from build123d import *

# Parameters (mm, degrees)
F0_R     = 3.175
F0_R_2   = 3.1994548284
F0_R_3   = 14.2875
F0_R_4   = 2.413
F0_R_5   = 13.97
F1_DEPTH = 6.35
F2_R     = 5.08


# Not quite as in the source:
# - a length typed as a fraction of an inch, garbled in the dataset ("3 / 203.2 mm" for 3/8 in), is restored


with BuildPart() as f1:
    # F0 (on Top) → F1 (new body)
    with BuildSketch(Plane.XY):
        Polygon((570.0438245296, 36.7193375349), (46.0845124741, 36.7193375349), (-39.5561754704, -42.6550139801), (-39.5561754704, -247.7606624651), (176.3438245296, -247.7606624651), (176.3438245296, -171.5606624651), (316.0438245296, -171.5606624651), (316.0438245296, -247.7606624651), (455.7438245296, -247.7606624651), (455.7438245296, -209.6606624651), (493.8438245296, -209.6606624651), (493.8438245296, -247.7606624651), (570.0438245296, -247.7606624651), align=None)
        with Locations((338.6971652508, -229.9806624651)):
            Circle(F0_R, mode=Mode.SUBTRACT)
        with Locations((373.4027445316, -229.9806624651)):
            Circle(F0_R, mode=Mode.SUBTRACT)
        with Locations((397.1410393715, -229.9806624651)):
            Circle(F0_R, mode=Mode.SUBTRACT)
        with Locations((425.3449738026, -229.9806624651)):
            Circle(F0_R_2, mode=Mode.SUBTRACT)
        with Locations((509.7217559814, -229.9806624651)):
            Circle(F0_R_2, mode=Mode.SUBTRACT)
        with Locations((529.0057063103, -229.9806624651)):
            Circle(F0_R_2, mode=Mode.SUBTRACT)
        with Locations((544.7416305542, -229.9806624651)):
            Circle(F0_R_2, mode=Mode.SUBTRACT)
        with Locations((508.030295372, -127.1675527096)):
            Circle(F0_R_3, mode=Mode.SUBTRACT)
        with Locations((272.5348336594, -89.2630653484)):
            Circle(F0_R_4, mode=Mode.SUBTRACT)
        with Locations((305.7173030479, -89.2630653484)):
            Circle(F0_R_4, mode=Mode.SUBTRACT)
        with Locations((289.1260683537, -72.6718306541)):
            Circle(F0_R_5, mode=Mode.SUBTRACT)
        with Locations((272.5348336594, -56.0805959599)):
            Circle(F0_R_4, mode=Mode.SUBTRACT)
        with Locations((305.7173030479, -56.0805959599)):
            Circle(F0_R_4, mode=Mode.SUBTRACT)
        with Locations((476.8743677037, -75.141350369)):
            Circle(F0_R_4, mode=Mode.SUBTRACT)
        with Locations((510.0568370922, -75.141350369)):
            Circle(F0_R_4, mode=Mode.SUBTRACT)
        with Locations((493.4656023979, -58.5501156747)):
            Circle(F0_R_5, mode=Mode.SUBTRACT)
        with Locations((476.8743677037, -41.9588809805)):
            Circle(F0_R_4, mode=Mode.SUBTRACT)
        with Locations((510.0568370922, -41.9588809805)):
            Circle(F0_R_4, mode=Mode.SUBTRACT)
        with Locations((290.5568880873, -31.5565178133)):
            Circle(F0_R, mode=Mode.SUBTRACT)
        with Locations((286.8396043777, 3.9247339591)):
            Circle(F0_R_3, mode=Mode.SUBTRACT)
    extrude(amount=F1_DEPTH)

    # F2
    f2_edges = [f1.edges().sort_by_distance(p)[0] for p in [
        (176.343825, -171.560662, 3.175),
        (316.043825, -171.560662, 3.175),
        (455.743825, -209.660662, 3.175),
        (493.843825, -209.660662, 3.175),
    ]]
    fillet(f2_edges, radius=F2_R)


solid = f1.part
Read the model definition and answer for the solid it produces. Units are mm, in the model's axes. Coordinates: 2 decimals unless noted, no trailing zeros. Order: outer loops, then holes, each group sorted by start corner. A loop starts at its lowest first (then second) coordinate and runs counter-clockwise, first axis right, second up. Notation, with made-up numbers: (83, 68.5) -> (110, 68.5) arc R22 ccw to (110, 78.5) -> close; hole circle Ø8 at (43, -37.75). An arc over 180 degrees is marked (long way). Answer as a JSON object with one key per item and string values.
1) Each of these flat-tipped pins is pushed along its axis until it touches: pin 1 (6 mm diameter, centred on x = 544.74, y = -229.98, fed in from -Z); pin 2 (2 mm diameter, centred on y = -25.5, z = 2.5, fed in from -X); pin 3 (3 mm diameter, centred on x = 471, z = 3.5, fed in from -Y); pin 4 (3 mm diameter, centred on x = 224, z = 3, fed in from -Y). Where does it stop, or does it pass through?
Model answer:
{"pin 1": "passes through", "pin 2": "stops at x = -22.13", "pin 3": "stops at y = -209.66", "pin 4": "stops at y = -171.56"}
2) A cutting plane is placed at B-B, the plane x = 223.5. Determine the outline of the cut face in (y, z).
Model answer:
{"outline": "(-171.56, 0) -> (36.72, 0) -> (36.72, 6.35) -> (-171.56, 6.35) -> close"}
3) The mould has two halves that part along X. Classify faces 1 (the face through (3.864, -2.412, 3.131)), 2 (the face through (482.38, -67.05, 3.13)), 3 (the face through (261, -104, 6.35)): released by +X, released by -X, zero draft, split by the parting line, or undercut.
Model answer:
{"face 1": "released by -X", "face 2": "undercut", "face 3": "zero draft"}
4) A cutting plane is placed at C-C, the plane y = 12. Determine the outline of the cut face in (x, z).
Model answer:
{"outline": "(19.41, 0) -> (275.05, 0) -> (275.05, 6.35) -> (19.41, 6.35) -> close; (298.63, 0) -> (570.04, 0) -> (570.04, 6.35) -> (298.63, 6.35) -> close"}
5) A cutting plane is placed at A-A, the plane y = -191. Determine the outline of the cut face in (x, z).
Model answer:
{"outline": "(-39.56, 0) -> (176.34, 0) -> (176.34, 6.35) -> (-39.56, 6.35) -> close; (316.04, 0) -> (570.04, 0) -> (570.04, 6.35) -> (316.04, 6.35) -> close"}
6) A cutting plane is placed at D-D, the plane z = 3. State how many separate pieces and enclosed holes the cut face has, plus the area to 3 significant figures.
Model answer:
{"separate pieces": "1", "enclosed holes": "20", "area": "155,000 mm²"}
7) Consider line 1 along X through (y, z) = (-214, 5.75); line 2 along Y through (x, z) = (268, 2.75); line 3 along X through (y, z) = (-188.5, 1). Determine where each line is inside the solid, lowest interval first. Write a range as from..to.
Model answer:
{"line 1": "x = -39.56..176.34, 316.04..455.8, 493.79..570.04", "line 2": "y = -171.56..36.72", "line 3": "x = -39.56..176.34, 316.04..570.04"}
